```python
from build123d import *

# Parameters (mm, degrees)
SKETCH1_R           = 1.5
BOSS_EXTRUDE1_DEPTH = 2.5


with BuildPart() as part:
    # Sketch1 → Boss-Extrude1 (new, symmetric)
    with BuildSketch(Plane.XY):
        with BuildLine():
            Line((1.083328706, 19.876336974), (1.083328706, 14.420285823))
            ThreePointArc((1.083328706, 14.420285823), (0.497542269, 13.006072261), (-0.916671294, 12.420285823))
            Line((-0.916671294, 12.420285823), (-6.916671294, 12.420285823))
            ThreePointArc((-6.916671294, 12.420285823), (-8.330884856, 11.834499385), (-8.916671294, 10.420285823))
            Line((-8.916671294, 10.420285823), (-8.916671294, -5.579714177))
            ThreePointArc((-8.916671294, -5.579714177), (-8.330884856, -6.993927739), (-6.916671294, -7.579714177))
            Line((-6.916671294, -7.579714177), (-0.916671294, -7.579714177))
            ThreePointArc((-0.916671294, -7.579714177), (0.497542269, -8.165500615), (1.083328706, -9.579714177))
            Line((1.083328706, -9.579714177), (1.083328706, -15.035765328))
            ThreePointArc((1.083328706, -15.035765328), (2.564962353, -18.588383827), (6.131767987, -20.035530686))
            add(Edge.make_bspline(
                [(6.131767987, -20.035530686), (9.248092377, -20.005338767), (12.570832777, -19.968565053), (16.083328706, -19.927626228)],
                knots=[0.046327938, 0.046327938, 0.046327938, 0.046327938, 0.128883425, 0.128883425, 0.128883425, 0.128883425], degree=3))
            Line((16.083328706, -19.927626228), (26.083328706, -19.927626228))
            Line((26.083328706, -19.927626228), (26.083328706, 24.768197874))
            Line((26.083328706, 24.768197874), (16.083328706, 24.768197874))
            add(Edge.make_bspline(
                [(16.083328706, 24.768197874), (12.570832777, 24.809136699), (9.248092377, 24.845910412), (6.131767987, 24.876102332)],
                knots=[0.046327938, 0.046327938, 0.046327938, 0.046327938, 0.128883425, 0.128883425, 0.128883425, 0.128883425], degree=3))
            ThreePointArc((6.131767987, 24.876102332), (2.564962353, 23.428955473), (1.083328706, 19.876336974))
        make_face()
        with Locations((13.083328706, 10.420285823)):
            Circle(SKETCH1_R, mode=Mode.SUBTRACT)
        with Locations((0.083328706, 2.420285823)):
            Circle(SKETCH1_R, mode=Mode.SUBTRACT)
        with Locations((13.083328706, -5.579714177)):
            Circle(SKETCH1_R, mode=Mode.SUBTRACT)
    extrude(amount=BOSS_EXTRUDE1_DEPTH, both=True)


solid = part.part
```
Can you work these out from the model? Positions are in its coordinate system, mm. A direction names the side the tool comes from. Coordinates: 2 decimals unless noted, no trailing zeros. Write each loop counter-clockwise with the first axis right and the second up, starting at its lowest first coordinate (ties: lowest second). Pieces come first, ordered by that corner, then holes. Notation, with made-up numbers: (87, 4.25) - (117, 4.25) arc R18 ccw to (117, 33.25) - close; hole circle Ø5 at (86.5, 49). An arc over 180 degrees is marked (long way). Return JSON: item names as keys, results as strings.
Q1. If we section it at C-C (z = -1.4): Count the separate pieces of the cut face and the enclosed holes in it, then the cut area to 3 significant figures.
Computed values:
{"separate pieces": "1", "enclosed holes": "3", "area": "1,290 mm2"}
Q2. On a 3-axis mill with a long thin cutter (end or side, diameter ignored), from which of +Z, -Z, +X, -X, +Y, -Y can I reach the whole of each face in a straight line? I mean faces 4 (the flat face through (-4, -7.58, 0)), 5 (the flat face through (1.083, 17, 0)), 6 (the flat face through (21, -19.928, 0)), 7 (the flat face through (21, 24.768, 0)). Say none if no direction works.
Computed values:
{"face 4": "+Z, -Z, -X, -Y", "face 5": "+Z, -Z, -X, +Y", "face 6": "+Z, -Z, +X, -Y", "face 7": "+Z, -Z, +X, +Y"}
Q3. I'm going to push flat-ended pins straight in: pin 1 Ø3 at (x, z) = (2, -1.5) entering from -Y; pin 2 Ø2.5 at (x, z) = (-3, 1) entering from +Y; pin 3 Ø1.8 at (x, y) = (13.08, 10.42) entering from +Z; pin 4 Ø2.5 at (y, z) = (16, 0.5) entering from -X. Where does each tip first touch, or does it pass through?
Computed values:
{"pin 1": "stops at y = -19.32", "pin 2": "stops at y = 12.42", "pin 3": "passes through", "pin 4": "stops at x = 1.08"}
Q4. Thinking about a two-plate mould opening in X: for faces 1 (the cylindrical face through (0.48, -8.15, 0.04)), 2 (the flat face through (12, 3, -2.5)), 3 (the cylindrical face through (11.585, -5.514, -0.035)), which applies, +X half, -X half, draft (parallel to the pull), parting line (faces both ways), or undercut?
Computed values:
{"face 1": "-X half", "face 2": "draft", "face 3": "undercut"}
Q5. If we section it at B-B (y = 19): Please give me the cut outline in (x, z), then the cut area to 3 significant figures.
Computed values:
{"outline": "(1.08, -2.5) - (26.08, -2.5) - (26.08, 2.5) - (1.08, 2.5) - close", "area": "125 mm2"}
Q6. If we section it at A-A (x = -6): Please give me the cut outline in (y, z).
Computed values:
{"outline": "(-7.58, -2.5) - (12.42, -2.5) - (12.42, 2.5) - (-7.58, 2.5) - close"}
Q7. Please list where these lines run through material, in increasing order: L1, parallel to Y at x = 13, z = -0.6; L2, parallel to Y at x = 24.5, z = 0.45; L3, parallel to Y at x = 6.5, z = 0.45. Write a range as from..to.
Computed values:
{"L1": "y = -19.96..-7.08, -4.08..8.92, 11.92..24.8", "L2": "y = -19.93..24.77", "L3": "y = -20.03..24.87"}
